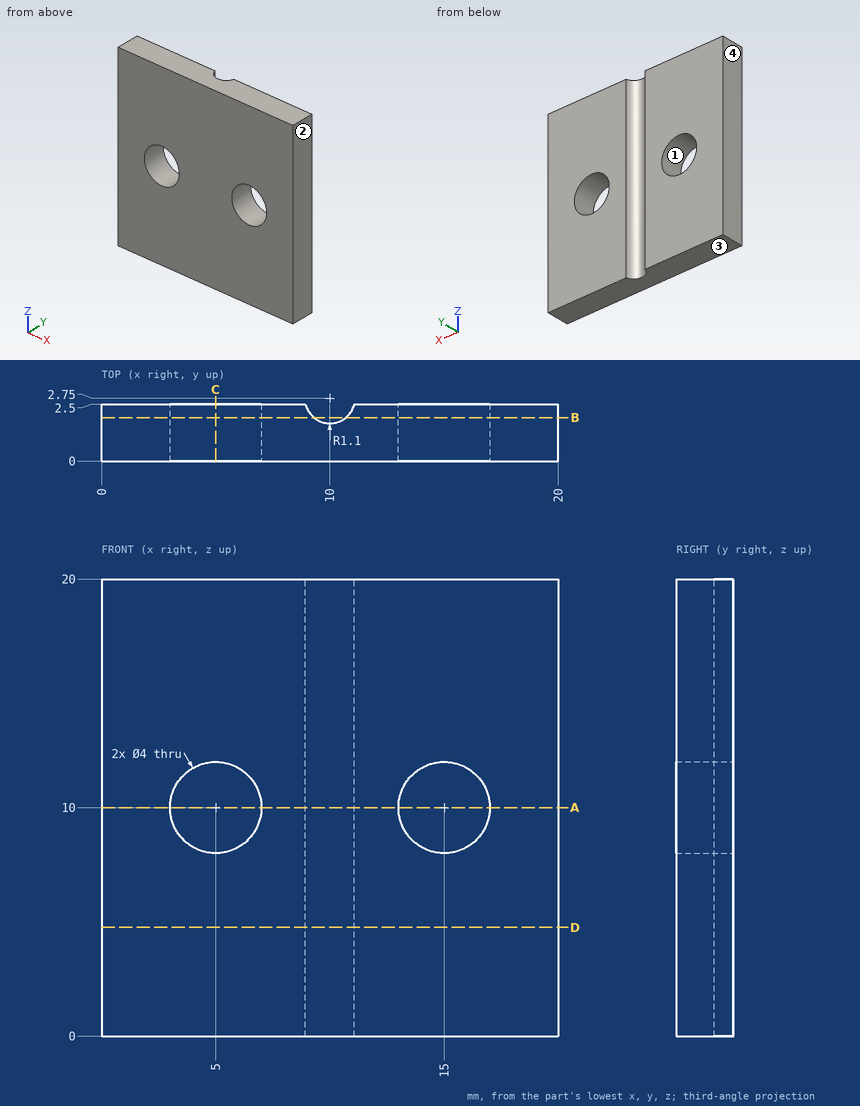
Check sheet for the drawn part. Datum: minimum x, y, z corner. Units: mm. Coordinates: 2 decimals unless noted, no trailing zeros. Write each loop counter-clockwise with the first axis right and the second up, starting at its lowest first coordinate (ties: lowest second). Pieces come first, ordered by that corner, then holes. Notation, with made-up numbers: M 23.25,41.5 L 42.25,41.5 A24 cw 42.25,80.5 Z; hole C -34.5,87 d3. An arc over 180 degrees is marked long. Use a Markdown table: item, result.
Q1. Sectioned sample at A-A, the plane z = 10. Record the boundary of the cut face in (x, y), plus the area to 3 significant figures.
Reply:
| item | result |
|---|---|
| outline | M 0,0 L 3,0 L 3,2.5 L 0,2.5 Z; M 7,0 L 13,0 L 13,2.5 L 11.07,2.5 A1.1 cw 8.93,2.5 L 7,2.5 Z; M 17,0 L 20,0 L 20,2.5 L 17,2.5 Z |
| area | 28.6 mm² |
Q2. Sectioned sample at D-D, the plane z = 4.75. Record the boundary of the cut face in (x, y).
Reply:
| item | result |
|---|---|
| outline | M 0,0 L 20,0 L 20,2.5 L 11.07,2.5 A1.1 cw 8.93,2.5 L 0,2.5 Z |
Q3. Sectioned sample at C-C, the plane x = 5. Record the boundary of the cut face in (y, z).
Reply:
| item | result |
|---|---|
| outline | M 0,0 L 2.5,0 L 2.5,8 L 0,8 Z; M 0,12 L 2.5,12 L 2.5,20 L 0,20 Z |
Q4. Draft check along X on the marked faces 1, 2, 3 and 4. Enter one of: +X half, -X half, draft (parallel to the pull), parting line (faces both ways), or undercut.
Reply:
| item | result |
|---|---|
| face 1 | undercut |
| face 2 | +X half |
| face 3 | draft |
| face 4 | -X half |
Q5. Sectioned sample at B-B, the plane y = 1.9. Record the boundary of the cut face in (x, z).
Reply:
| item | result |
|---|---|
| outline | M 0,0 L 9.3,0 L 9.3,20 L 0,20 Z; M 10.7,0 L 20,0 L 20,20 L 10.7,20 Z; hole C 5,10 d4; hole C 15,10 d4 |
Q6. Thickness scan on line 1 (X direction, y = 1, z = 10); line 2 (Z direction, x = 15, y = 1.7); line 3 (X direction, y = 0.35, z = 11.5). Record the ranges inside material, lowest first.
Reply:
| item | result |
|---|---|
| line 1 | x = 0 to 3, 7 to 13, 17 to 20 |
| line 2 | z = 0 to 8, 12 to 20 |
| line 3 | x = 0 to 3.68, 6.32 to 13.68, 16.32 to 20 |
